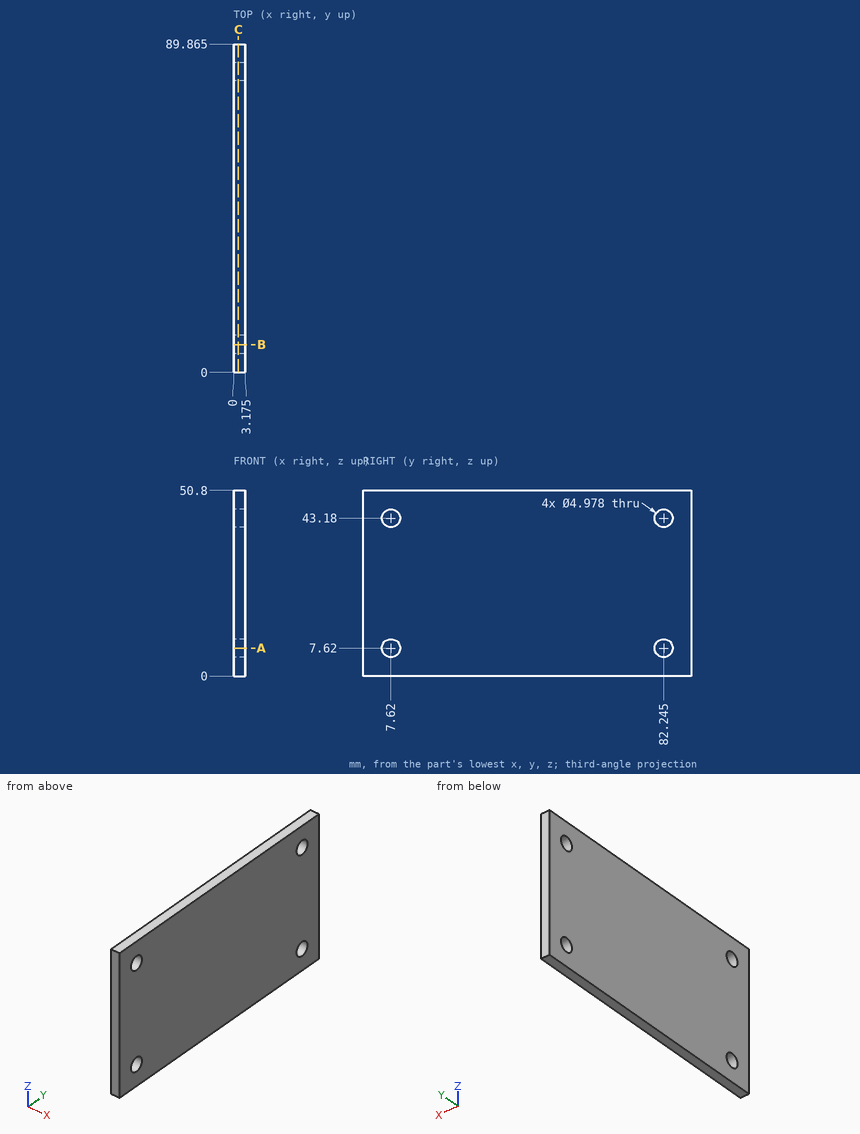
Input: dimensioned drawing with shaded views. Units: mm. Origin: part minimum x, y, z. Coordinates: 2 decimals unless noted, no trailing zeros. Loops run counter-clockwise (first coordinate to the right, second up) from the corner with the lowest first, then second, coordinate; pieces in that order, holes last. Notation, with made-up numbers: (16, 49.5) -> (34, 49.5) arc R30 cw to (34, 82.5) -> close; hole circle Ø5 at (-29.5, 66.5). An arc over 180 degrees is marked (long way). One line per item, written item: value. Start each with the question number.
Q1. Section query B-B, the plane y = 7.62. Return the cut outline in (x, z) (1 decimal), and give its area (3 significant figures).
Q2. Line query: line 1 along Z through (x, y) = (1.35, 7.62); line 2 along Y through (x, z) = (1.05, 43.18) (1 decimal); line 3 along Z through (x, y) = (0.75, 8). Output: solid intervals per line, ascending.
Q3. Section query C-C, the plane x = 1.3. Return the cut outline in (y, z) (1 decimal).
Q4. Section query A-A, the plane z = 7.62. Return the cut outline in (x, y) (1 decimal), and give its area (3 significant figures).
Results:
1. outline: (0, 0) -> (3.2, 0) -> (3.2, 5.1) -> (0, 5.1) -> close; (0, 10.1) -> (3.2, 10.1) -> (3.2, 40.7) -> (0, 40.7) -> close; (0, 45.7) -> (3.2, 45.7) -> (3.2, 50.8) -> (0, 50.8) -> close
1. area: 130 mm^2
2. line 1: 0 to 5.13, 10.11 to 40.69, 45.67 to 50.8
2. line 2: 0 to 5.1, 10.1 to 79.8, 84.7 to 89.9
2. line 3: 0 to 5.16, 10.08 to 40.72, 45.64 to 50.8
3. outline: (0, 0) -> (89.9, 0) -> (89.9, 50.8) -> (0, 50.8) -> close; hole circle Ø5 at (7.6, 7.6); hole circle Ø5 at (7.6, 43.2); hole circle Ø5 at (82.2, 7.6); hole circle Ø5 at (82.2, 43.2)
4. outline: (0, 0) -> (3.2, 0) -> (3.2, 5.1) -> (0, 5.1) -> close; (0, 10.1) -> (3.2, 10.1) -> (3.2, 79.8) -> (0, 79.8) -> close; (0, 84.7) -> (3.2, 84.7) -> (3.2, 89.9) -> (0, 89.9) -> close
4. area: 254 mm^2
